Autodesk Inventor part; units mm, degrees
ref_plane "YZ Plane" through (0, 0, 0) normal (1, 0, 0) x (0, 1, 0)
ref_plane "XZ Plane" through (0, 0, 0) normal (0, 1, 0) x (-1, 0, 0)
ref_plane "XY Plane" through (0, 0, 0) normal (0, 0, 1) x (1, 0, 0)
sketch "Sketch1" plane through (0, 0, 0) normal (0, 1, 0) x (-1, 0, 0)
  line L0 (0, 0) -> (94, 0)
  line L1 (94, 0) -> (94, -94)
  line L2 (94, -94) -> (0, -94)
  line L3 (0, -94) -> (0, 0)
  line L4 (84, -10) -> (10, -10)
  line L5 (10, -10) -> (10, -84)
  line L6 (10, -84) -> (84, -84)
  line L7 (84, -84) -> (84, -10)
  line L8 (47, 0) -> (47, -10) construction
  line L9 (10, -47) -> (0, -47) construction
  dimension "d1" = 74
  dimension "d3" = 10
extrude "Extrusion1" add sketch "Sketch1" along normal blind 50
sketch "Sketch2" plane through (-94, 0, 0) normal (0, 0, 1) x (1, 0, 0)
  line L0 (10, 50) -> (84, 50) construction
  line L1 (16, 50) -> (16, 34) construction
  line L2 (16, 16) -> (16, 0) construction
  line L3 (16, 34) -> (0, 34) construction
  line L4 (0, 0) -> (0, 50) construction
  line L5 (78, 50) -> (78, 34) construction
  line L6 (78, 34) -> (94, 34) construction
  line L7 (94, 0) -> (94, 50) construction
  line L8 (94, 16) -> (78, 16) construction
  line L9 (78, 16) -> (78, 0) construction
  circle A0 centre (16, 34) radius 2
  circle A1 centre (78, 34) radius 2
  circle A2 centre (78, 16) radius 2
  circle A3 centre (16, 16) radius 2
  line L10 (0, 0) -> (94, 0) construction
  dimension "boarder_to_hole" = 16
  dimension "d7" = 4
extrude "Extrusion2" cut sketch "Sketch2" against normal up to surface (94 mm away)
sketch "Sketch3" plane through (0, 0, 0) normal (1, 0, 0) x (0, 0, -1)
  line L0 (0, 50) -> (60.8888, 50) construction
  line L1 (16, 50) -> (16, 34) construction
  line L2 (16, 16) -> (16, 0) construction
  line L3 (16, 34) -> (0, 34) construction
  line L4 (0, 0) -> (0, 50) construction
  line L5 (78, 50) -> (78, 34) construction
  line L6 (78, 34) -> (94, 34) construction
  line L7 (94, 0) -> (94, 49.9084) construction
  line L8 (94, 16) -> (78, 16) construction
  line L9 (78, 16) -> (78, 0) construction
  circle A0 centre (16, 34) radius 2
  circle A1 centre (78, 34) radius 2
  circle A2 centre (78, 16) radius 2
  circle A3 centre (16, 16) radius 2
  line L10 (0, 0) -> (94, 0) construction
  line L11 (0, 50) -> (94, 50)
  dimension "d10" = 16
  dimension "d13" = 4
extrude "Extrusion3" cut sketch "Sketch3" against normal up to surface (94 mm away)
fillet "Fillet1" radius 3 4 edges at (0, 25, 0) (-94, 25, 0) (-94, 25, -94) (0, 25, -94)
equation "\"d3\" = square_thickness"
equation "\"d7\" = screw_size"
equation "\"d10\" = boarder_to_hole"
equation "\"d13\" = screw_size"
properties part number "centerlegg_mounting_bracket"
The model under review builds one solid part; all positions refer to its coordinate system, in mm. A direction names the side the tool comes from. Round coordinates to 2 decimals unless told otherwise and drop trailing zeros. Order: outer loops, then holes, each group sorted by start corner. A loop starts at its lowest first (then second) coordinate and runs counter-clockwise, first axis right, second up. Notation, with made-up numbers: (2, 48) -> (18, 48) arc R23 cw to (18, 64) -> close; hole circle Ø4 at (61.5, 73). An arc over 180 degrees is marked (long way). Write item = value, one per line. Start each with the question number.
Item 1: For line 1 along Y through (x, z) = (-6.5, -78); line 2 along X through (y, z) = (27, -66), list the stretches that pass through material, from the lowest coordinate up.
Item 2: Consider section D-D on y = 4.5. Write out the cut boundary in (x, z), plus the area to 3 significant figures.
Item 3: Consider section A-A on z = -78. Write out the cut boundary in (x, y).
Item 4: Consider section B-B on x = -40.5. Write out the cut boundary in (y, z).
Item 5: Consider section C-C on z = -48.5. Write out the cut boundary in (x, y).
Item 6: For faces 1 (the face through (-48, 25, -10)), 2 (the face through (-16, 18, -89)), list the 3-axis set-ups (+Z, -Z, +X, -X, +Y, -Y) from which the entire face can be reached by the end or side of a thin tool; tool diameter is ignored.
Item 7: Mouldability with a two-part tool opening along Y and no side actions: class faces 3 (the face through (-0.9, 25.35, -0.86)), 4 (the face through (-76.092, 16.601, -88.93)), 5 (the face through (-5, 50, -46)) as released by +Y, released by -Y, zero draft, split by the parting line, or undercut.
Conclusion:
q1.line_1 = 0 to 14, 18 to 32, 36 to 50
q1.line_2 = -94 to -84, -10 to 0
q2.outline = (-94, -91) arc R3 ccw to (-91, -94) -> (-3, -94) arc R3 ccw to (0, -91) -> (0, -3) arc R3 ccw to (-3, 0) -> (-91, 0) arc R3 ccw to (-94, -3) -> close; hole (-84, -84) -> (-10, -84) -> (-10, -10) -> (-84, -10) -> close
q2.area = 3,350 mm2
q3.outline = (-94, 0) -> (-84, 0) -> (-84, 14) -> (-94, 14) -> close; (-94, 18) -> (-84, 18) -> (-84, 32) -> (-94, 32) -> close; (-94, 36) -> (-84, 36) -> (-84, 50) -> (-94, 50) -> close; (-10, 0) -> (0, 0) -> (0, 14) -> (-10, 14) -> close; (-10, 18) -> (0, 18) -> (0, 32) -> (-10, 32) -> close; (-10, 36) -> (0, 36) -> (0, 50) -> (-10, 50) -> close
q4.outline = (0, -94) -> (50, -94) -> (50, -84) -> (0, -84) -> close; (0, -10) -> (50, -10) -> (50, 0) -> (0, 0) -> close
q5.outline = (-94, 0) -> (-84, 0) -> (-84, 50) -> (-94, 50) -> close; (-10, 0) -> (0, 0) -> (0, 50) -> (-10, 50) -> close
q6.face_1 = +Y, -Y
q6.face_2 = +Z, -Z
q7.face_3 = zero draft
q7.face_4 = undercut
q7.face_5 = released by +Y
